from build123d import *

# Parameters (mm, degrees)
BOSS_EXTRUDE1_DEPTH = 7.5
CHAMFER1_SIZE       = 2.5
SKETCH2_R           = 16.5
BOSS_EXTRUDE2_DEPTH = 5
BOSS_EXTRUDE3_DEPTH = 5
FILLET1_R           = 1
SKETCH4_R           = 5
CUT_EXTRUDE1_DEPTH  = 10
SKETCH5_R           = 5
BOSS_EXTRUDE4_DEPTH = 10


with BuildPart() as part:
    # Sketch1 → Boss-Extrude1 (new body, symmetric)
    with BuildSketch(Plane.XY):
        with BuildLine():
            ThreePointArc((85, -15), (99.994474711, 0.407097217), (84.186105477, 14.977902914))
            ThreePointArc((84.186105477, 14.977902914), (0.617423728, 13.934366249), (-82.746539792, 19.872642429))
            ThreePointArc((-82.746539792, 19.872642429), (-104.804980291, 2.786172224), (-88.316875687, -19.723040731))
            ThreePointArc((-88.316875687, -19.723040731), (-1.428818786, -25.787629696), (85, -15))
        make_face()
    extrude(amount=BOSS_EXTRUDE1_DEPTH, both=True)

    # Chamfer1
    chamfer1_edges = [part.edges().sort_by_distance(p)[0] for p in [
        (99.994474711, 0.407097217, 7.5),
        (0.617423728, 13.934366249, 7.5),
        (-104.804980291, 2.786172224, 7.5),
        (-1.428818786, -25.787629696, 7.5),
        (-104.804980291, 2.786172224, -7.5),
        (0.617423728, 13.934366249, -7.5),
        (99.994474711, 0.407097217, -7.5),
        (-1.428818786, -25.787629696, -7.5),
    ]]
    chamfer(chamfer1_edges, length=CHAMFER1_SIZE)

    # Sketch2 → Boss-Extrude2 (add)
    with BuildSketch(Plane.XY.offset(7.5)):
        with Locations((-85, 0)):
            Circle(SKETCH2_R)
    extrude(amount=BOSS_EXTRUDE2_DEPTH)

    # Sketch3 → Boss-Extrude3 (add)
    with BuildSketch(Plane.XY.offset(12.5)):
        with BuildLine():
            Line((-70.454369396, 8.397923745), (-85, 0))
            Line((-85, 0), (-68.20415251, 0))
            ThreePointArc((-68.20415251, 0), (-65.824092489, 1.173715713), (-65.306375031, 3.776457135))
            Line((-65.306375031, 3.776457135), (-66.056591917, 6.576304669))
            ThreePointArc((-66.056591917, 6.576304669), (-67.806319099, 8.571486131), (-70.454369396, 8.397923745))
        make_face()
        with BuildLine():
            Line((-72.518252849, -11.238615615), (-85, 0))
            Line((-85, 0), (-79.809797691, -15.973800202))
            ThreePointArc((-79.809797691, -15.973800202), (-77.95804872, -17.874673692), (-75.322711037, -17.562760922))
            Line((-75.322711037, -17.562760922), (-72.891727563, -15.984061795))
            ThreePointArc((-72.891727563, -15.984061795), (-71.534892666, -13.703427379), (-72.518252849, -11.238615615))
        make_face()
        with BuildLine():
            Line((-91.831486626, -15.343770181), (-85, 0))
            Line((-85, 0), (-98.588126054, -9.872351454))
            ThreePointArc((-98.588126054, -9.872351454), (-99.823742272, -12.220871592), (-98.71273147, -14.630840322))
            Line((-98.71273147, -14.630840322), (-96.460084172, -16.454998137))
            ThreePointArc((-96.460084172, -16.454998137), (-93.871786907, -17.040670013), (-91.831486626, -15.343770181))
        make_face()
        with BuildLine():
            Line((-101.70383808, 1.755644127), (-85, 0))
            Line((-85, 0), (-98.588126054, 9.872351454))
            ThreePointArc((-98.588126054, 9.872351454), (-101.203527845, 10.321759676), (-103.15222309, 8.52040432))
            Line((-103.15222309, 8.52040432), (-104.190993969, 5.814313662))
            ThreePointArc((-104.190993969, 5.814313662), (-103.948173183, 3.171714119), (-101.70383808, 1.755644127))
        make_face()
        with BuildLine():
            Line((-88.49205305, 16.428817924), (-85, 0))
            Line((-85, 0), (-79.809797691, 15.973800202))
            ThreePointArc((-79.809797691, 15.973800202), (-80.190588674, 18.600069896), (-82.505959371, 19.896739789))
            Line((-82.505959371, 19.896739789), (-85.400602379, 20.048441601))
            ThreePointArc((-85.400602379, 20.048441601), (-87.838828145, 19.000897142), (-88.49205305, 16.428817924))
        make_face()
    extrude(amount=-BOSS_EXTRUDE3_DEPTH)

    # Fillet1
    fillet1_edges = [part.edges().sort_by_distance(p)[0] for p in [
        (-77.95804872, -17.874673692, 12.5),
        (-79.855508642, -15.83311636, 12.5),
        (-74.1072193, -16.773411359, 12.5),
        (-71.534892666, -13.703427379, 12.5),
        (-72.628181614, -11.13963531, 12.5),
        (-85.863543278, -16.477387323, 12.5),
        (-99.823742272, -12.220871592, 12.5),
        (-98.468453231, -9.785404059, 12.5),
        (-97.586407821, -15.542919229, 12.5),
        (-93.871786907, -17.040670013, 12.5),
        (-91.771320618, -15.208635116, 12.5),
        (-100.937776134, -4.270514244, 12.5),
        (-101.203527845, 10.321759676, 12.5),
        (-98.468453231, 9.785404059, 12.5),
        (-103.67160853, 7.167358991, 12.5),
        (-103.948173183, 3.171714119, 12.5),
        (-101.556724677, 1.740181886, 12.5),
        (-93.986544078, 13.838064371, 12.5),
        (-80.190588674, 18.600069896, 12.5),
        (-79.855508642, 15.83311636, 12.5),
        (-83.953280875, 19.972590695, 12.5),
        (-87.838828145, 19.000897142, 12.5),
        (-88.461297974, 16.284126668, 12.5),
        (-74.616213548, 12.822908364, 12.5),
        (-65.824092489, 1.173715713, 12.5),
        (-68.352076255, 0, 12.5),
        (-65.681483474, 5.176380902, 12.5),
        (-67.806319099, 8.571486131, 12.5),
        (-70.582475117, 8.323961872, 12.5),
        (-69.595922963, -5.913071167, 12.5),
    ]]
    fillet(fillet1_edges, radius=FILLET1_R)

    # Sketch4 → Cut-Extrude1 (cut)
    with BuildSketch(Plane.XY.offset(7.5)):
        with Locations((85.615305239, 0)):
            Circle(SKETCH4_R)
    extrude(amount=-CUT_EXTRUDE1_DEPTH, mode=Mode.SUBTRACT)

    # Sketch5 → Boss-Extrude4 (add)
    with BuildSketch(Plane(origin=(0, 0, -7.5), x_dir=(-1, 0, 0), z_dir=(0, 0, -1))):
        with Locations((85, 0)):
            Circle(SKETCH5_R)
    extrude(amount=BOSS_EXTRUDE4_DEPTH)


solid = part.part
CAD build for the part. Positions are in the model's coordinates, mm. A direction names the side the tool comes from. Round coordinates to 2 decimals unless told otherwise and drop trailing zeros. Use one line per item in the form item = value.
Q1. Flat gauge pins, fed straight in: P1, Ø6, axis at x = -47.5, y = 13.5, coming from the -Z side; P2, Ø2, axis at y = -11, z = -9, coming from the -X side; P3, Ø3, axis at x = 85, y = -2.5, coming from the +Z side; P4, Ø3, axis at y = -2, z = -13.5, coming from the -X side. Where does each tip first touch, or does it go through?
Recorded:
P1 = -7.5
P2 = through
P3 = -2.5
P4 = -89.97
Q2. Two-plate mould, pull along Z, no slides. Class faces 6 (the cylindrical face through (-93.91, -17.05, 9.53)), 7 (the flat face through (-101, -5, 7.5)), 8 (the flat face through (-97, -14, 7.5)): +Z half, -Z half, draft (parallel to the pull), parting line (faces both ways), or undercut.
Recorded:
face_6 = draft
face_7 = +Z half
face_8 = undercut
Q3. Which spindle directions (+Z, -Z, +X, -X, +Y, -Y) get a long thin tool onto all of the face, cutting with end or side? Do faces 1 (the cylindrical face through (1.8, 13.9, 0.1)), 2 (the cylindrical face through (-99.822, -12.182, 9.528)), 3 (the cylindrical face through (-89.619, -1.915, -12.43)), 4 (the cylindrical face through (-77.994, -17.862, 9.528)), 5 (the flat face through (86, 0, -2.5)). Say none if no direction does.
Recorded:
face_1 = +Z, -Z, +Y
face_2 = +Z, -X
face_3 = -Z
face_4 = +Z, -Y
face_5 = +Z
Q4. Probe L1, parallel to Z at x = 37.5, y = -1.5; L2, parallel to Z at x = -88, y = -5; L3, parallel to X at y = 0.5, z = -10. List the from-to ranges inside material, lowest first.
Recorded:
L1 = -7.5 to 7.5
L2 = -7.5 to 12.5
L3 = -89.97 to -80.03
